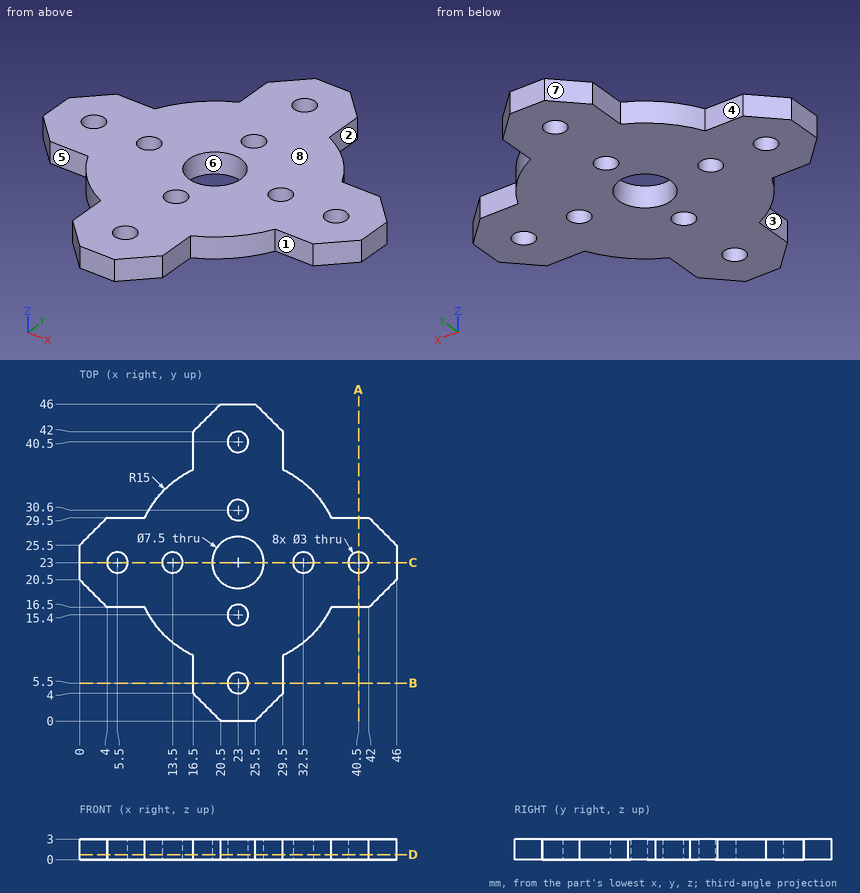
Geometry check sheet. Reference: drawing and pictorial views, mm from the part's lowest x, y, z. A direction names the side the tool comes from. Coordinates: 2 decimals unless noted, no trailing zeros. Order: outer loops, then holes, each group sorted by start corner. A loop starts at its lowest first (then second) coordinate and runs counter-clockwise, first axis right, second up. Notation, with made-up numbers: (-36, 20) - (-2, 20) arc R26 ccw to (-2, 45) - close; hole circle Ø11 at (-6.5, 29). An arc over 180 degrees is marked (long way). One line per item, written item: value.
(1) Depth check by flat-ended pin: pin 1 Ø1.5 at (y, z) = (13, 1) entering from +X; pin 2 Ø1.5 at (y, z) = (40, 2) entering from +X; pin 3 Ø2.5 at (x, y) = (13.5, 23) entering from +Z; pin 4 Ø1.5 at (x, z) = (5.5, 2) entering from -Y. Enter the tip coordinate at first touch or a pass-through.
Data:
pin 1: stops at x = 34.81
pin 2: stops at x = 29.5
pin 3: passes through
pin 4: stops at y = 16.5
(2) Sectioned sample at D-D (z = 0.75). Count the separate pieces of the cut face and the enclosed holes in it, and give its area (3 significant figures).
Data:
separate pieces: 1
enclosed holes: 9
area: 983 mm^2
(3) Release check for a two-part mould opening along Y. For the marked faces 5, 6, 7 and 8 record: +Y half, -Y half, draft (parallel to the pull), parting line (faces both ways), or undercut.
Data:
face 5: -Y half
face 6: undercut
face 7: +Y half
face 8: draft
(4) Access from +Z, -Z, +X, -X, +Y, -Y to the whole of each face (thin tool, end or side, straight path). Record for the marked faces 1, 2, 3 and 4.
Data:
face 1: +Z, -Z, +X, -Y
face 2: +Z, -Z, +X, +Y
face 3: +Z, -Z, -X, -Y
face 4: +Z, -Z, -X, +Y
(5) Sectioned sample at C-C (y = 23). Enter the section's corners in (x, z).
Data:
outline: (0, 0) - (4, 0) - (4, 3) - (0, 3) - close; (7, 0) - (12, 0) - (12, 3) - (7, 3) - close; (15, 0) - (19.25, 0) - (19.25, 3) - (15, 3) - close; (26.75, 0) - (31, 0) - (31, 3) - (26.75, 3) - close; (34, 0) - (39, 0) - (39, 3) - (34, 3) - close; (42, 0) - (46, 0) - (46, 3) - (42, 3) - close
(6) Thickness scan on probe 1 along Y at (x, z) = (23, 0.95); probe 2 along Y at (x, z) = (5.5, 1.2); probe 3 along X at (y, z) = (41, 0.9). Record the ranges inside material, lowest first. Write a range as from..to.
Data:
probe 1: y = 0..4, 7..13.9, 16.9..19.25, 26.75..29.1, 32.1..39, 42..46
probe 2: y = 16.5..21.5, 24.5..29.5
probe 3: x = 16.5..21.59, 24.41..29.5
(7) Sectioned sample at A-A (x = 40.5). Enter the section's corners in (y, z).
Data:
outline: (16.5, 0) - (21.5, 0) - (21.5, 3) - (16.5, 3) - close; (24.5, 0) - (29.5, 0) - (29.5, 3) - (24.5, 3) - close
